Build history of the part. All positions in model axes, mm. A direction names the side the tool comes from. Round coordinates to 2 decimals unless told otherwise and drop trailing zeros. Write each loop counter-clockwise with the first axis right and the second up, starting at its lowest first coordinate (ties: lowest second). Pieces come first, ordered by that corner, then holes.
from build123d import *

# Parameters (mm, degrees)
F0_R     = 15.875
F0_R_2   = 4.7625
F1_DEPTH = 12.7
F2_W     = 39.643920958
F2_H     = 19.4333904848
F3_DEPTH = 12.701
F4_R     = 1.89865
F5_DEPTH = 14.2885
F7_R     = 4.7625
F8_DEPTH = 9.525


# Not quite as in the source:
# - a length typed as a fraction of an inch, garbled in the dataset ("3 / 203.2 mm" for 3/8 in), is restored


with BuildPart() as f1:
    # F0 (on Right) → F1 (new body)
    with BuildSketch(Plane.YZ):
        Circle(F0_R)
        Circle(F0_R_2, mode=Mode.SUBTRACT)
    extrude(amount=F1_DEPTH)

    # F2 (on face) → F3 (cut, through all)
    with BuildSketch(Plane.YZ.offset(12.7)):
        with Locations((-1.8631611019, 8.1291952424)):
            Rectangle(F2_W, F2_H)
    extrude(amount=-F3_DEPTH, mode=Mode.SUBTRACT)

    # F4 (on face) → F5 (cut, through all)
    with BuildSketch(Plane.XY.offset(-1.5875)):
        with Locations((6.35, -10.1427768123)):
            Circle(F4_R)
        with Locations((6.35, 10.1427768123)):
            Circle(F4_R)
    extrude(amount=-F5_DEPTH, mode=Mode.SUBTRACT)

    # F7 (on offset) → F8 (cut)
    with BuildSketch(Plane.XY.offset(-15.875)):
        with Locations((6.35, 10.1427768123)):
            Circle(F7_R)
        with Locations((6.35, -10.1427768123)):
            Circle(F7_R)
    extrude(amount=F8_DEPTH, mode=Mode.SUBTRACT)


solid = f1.part
1) Pin check, flat tips, straight feed: pin 1 Ø2.5 at (x, y) = (6.35, -10.14) entering from +Z; pin 2 Ø3 at (x, y) = (8.5, -9) entering from -Z; pin 3 Ø4 at (x, y) = (4, 5) entering from -Z; pin 4 Ø1.5 at (x, y) = (6.5, 3.5) entering from +Z. Stop position of each tip, or through.
Results:
pin 1: passes through
pin 2: stops at z = -6.35
pin 3: stops at z = -15.59
pin 4: stops at z = -2.15
2) Mould opens along Y. For faces 3 (the cylindrical face through (6.26, -0.08, -4.76)), 4 (the flat face through (0, 0, -9)), 5 (the cylindrical face through (6.26, -0.33, -15.87)) say: released by +Y, released by -Y, zero draft, split by the parting line, or undercut.
Results:
face 3: undercut
face 4: zero draft
face 5: split by the parting line
3) Slice it at A-A (x = 6.35). Count the separate pieces of the cut face and the enclosed holes in it, plus the area to 3 significant figures.
Results:
separate pieces: 3
enclosed holes: 0
area: 188 mm2
4) Slice it at B-B (y = 7). Write the cut outline in (x, z).
Results:
outline: (0, -14.25) - (2.77, -14.25) - (2.77, -6.35) - (9.93, -6.35) - (9.93, -14.25) - (12.7, -14.25) - (12.7, -1.59) - (0, -1.59) - close
5) Which spindle directions (+Z, -Z, +X, -X, +Y, -Y) get a long thin tool onto all of the face, cutting with end or side? Do faces 1 (the cylindrical face through (6.167, 5.384, -9.749)), 2 (the flat face through (12.7, 0, -9)). Say none if no direction does.
Results:
face 1: -Z
face 2: +Z, -Z, +X, +Y, -Y
6) Wall check: L1, parallel to Y at x = 6.35, z = -3.35; L2, parallel to Y at x = 6.35, z = -12.25; L3, parallel to Y at x = 3.5, z = -3.5. Give the ranges that are in metal, low to high.
Results:
L1: y = -15.52 to -12.04, -8.24 to -3.39, 3.39 to 8.24, 12.04 to 15.52
L2: y = -5.38 to 5.38
L3: y = -15.48 to -3.23, 3.23 to 15.48
